```python
from build123d import *

# Parameters (mm, degrees)
CROQUIS1_R              = 3.5
CROQUIS1_R_2            = 0.99
SALIENTE_EXTRUIR1_DEPTH = 5
CORTAR_EXTRUIR1_START   = -5
CORTAR_EXTRUIR1_DEPTH   = 5
MATRIZC1_COUNT          = 14


with BuildPart() as part:
    # Croquis1 → Saliente-Extruir1 (new body)
    with BuildSketch(Plane.XY):
        Circle(CROQUIS1_R)
        Circle(CROQUIS1_R_2, mode=Mode.SUBTRACT)
    extrude(amount=SALIENTE_EXTRUIR1_DEPTH)

    # Croquis2 → Cortar-Extruir1 (cut)
    with BuildSketch(Plane.XY.offset(5).offset(CORTAR_EXTRUIR1_START)):
        with BuildLine():
            ThreePointArc((0.516991774, 3.461606492), (-0.284402129, 3.488425924), (-1.070868948, 3.332152412))
            ThreePointArc((-1.070868948, 3.332152412), (-0.501013204, 2.913608412), (-0.354709173, 2.221864398))
            ThreePointArc((-0.354709173, 2.221864398), (-0.18282994, 2.242559523), (-0.009868326, 2.249978359))
            ThreePointArc((-0.009868326, 2.249978359), (0.022456296, 2.956285494), (0.516991774, 3.461606492))
        make_face()
    cortar_extruir1 = extrude(amount=CORTAR_EXTRUIR1_DEPTH, mode=Mode.SUBTRACT)

    # MatrizC1: Cortar-Extruir1 ×14 about axis
    matrizc1_axis = Axis((0, 0, 0), (0, 0, 1))
    for i in range(1, MATRIZC1_COUNT):
        add(cortar_extruir1.rotate(matrizc1_axis, i * 360 / MATRIZC1_COUNT), mode=Mode.SUBTRACT)


solid = part.part
```
Check sheet for the modelled part. Datum: model origin and axes. Units: mm. Round coordinates to 2 decimals unless told otherwise and drop trailing zeros. Order: outer loops, then holes, each group sorted by start corner. A loop starts at its lowest first (then second) coordinate and runs counter-clockwise, first axis right, second up. Notation, with made-up numbers: M 3,36 L 9,36 A21 cw 9,61 Z; hole C 38,-29 d5. An arc over 180 degrees is marked long. Answer in a Markdown table with one row per item.
(1) Section check B-B on x = 2.75. Record the boundary of the cut face in (y, z).
Findings:
| item | result |
|---|---|
| outline | M -1.43,0 L -0.6,0 L -0.6,5 L -1.43,5 Z; M -0.21,0 L 0.65,0 L 0.65,5 L -0.21,5 Z; M 1.16,0 L 1.85,0 L 1.85,5 L 1.16,5 Z |
(2) Gauge pin test, flat ends, axial feed: pin 1 (1 mm diameter, centred on x = -1.5, z = 1.5, fed in from -Y); pin 2 (2 mm diameter, centred on x = 2.5, y = -1.5, fed in from -Z). Record the tip position at first contact, or that the pin passes through.
Findings:
| item | result |
|---|---|
| pin 1 | stops at y = -2.89 |
| pin 2 | stops at z = 0 |
(3) Draft check along Y on faces 1 (the cylindrical face through (-2.31, -1.82, 2.46)), 2 (the flat face through (1, 1, 0)). Enter one of: +Y half, -Y half, draft (parallel to the pull), parting line (faces both ways), or undercut.
Findings:
| item | result |
|---|---|
| face 1 | undercut |
| face 2 | draft |
(4) Material ranges on line 1 along Y through (x, z) = (-2.5, 3.55); line 2 along Y through (x, z) = (2.75, 2.5); line 3 along X through (y, z) = (3, 4), recorded low to high. Write a range as from..to.
Findings:
| item | result |
|---|---|
| line 1 | y = -1.86..-0.96, -0.63..0.21, 0.51..1.41 |
| line 2 | y = -1.43..-0.6, -0.21..0.65, 1.16..1.85 |
| line 3 | x = -1.22..-0.56, 0.04..0.78 |
(5) Section check A-A on y = 0. Record the boundary of the cut face in (x, z), plus the area to 3 significant figures.
Findings:
| item | result |
|---|---|
| outline | M -3.24,0 L -0.99,0 L -0.99,5 L -3.24,5 Z; M 0.99,0 L 3.24,0 L 3.24,5 L 0.99,5 Z |
| area | 22.5 mm^2 |
(6) Section check C-C on x = 0.25. Record the boundary of the cut face in (y, z), plus the area to 3 significant figures.
Findings:
| item | result |
|---|---|
| outline | M -2.24,0 L -0.96,0 L -0.96,5 L -2.24,5 Z; M 0.96,0 L 3.28,0 L 3.28,5 L 0.96,5 Z |
| area | 18.0 mm^2 |
